from build123d import *

# Parameters (mm, degrees)
BOSS_EXTRUDE1_DEPTH = 4.5
BOSS_EXTRUDE2_START = 0.5
BOSS_EXTRUDE2_DEPTH = 0.5
FILLET1_R           = 0.5
FILLET2_R           = 0.1


with BuildPart() as part:
    # Sketch1 → Boss-Extrude1 (new body)
    with BuildSketch(Plane(origin=(0, 0, 0), x_dir=(1, 0, 0), z_dir=(0, 1, 0))):
        with BuildLine():
            Line((-2, 1.8), (2, 1.8))
            ThreePointArc((2, 1.8), (3.8, 0), (2, -1.8))
            Line((2, -1.8), (-2, -1.8))
            ThreePointArc((-2, -1.8), (-3.8, 0), (-2, 1.8))
        make_face()
    extrude(amount=BOSS_EXTRUDE1_DEPTH)

    # Sketch2 → Boss-Extrude2 (add)
    # profile 1 of 2: a face of its own
    with BuildSketch(Plane.XZ.offset(BOSS_EXTRUDE2_START)):
        with BuildLine():
            Line((-2, -2.4), (2, -2.4))
            ThreePointArc((2, -2.4), (4.4, 0), (2, 2.4))
            Line((2, 2.4), (-2, 2.4))
            ThreePointArc((-2, 2.4), (-4.4, 0), (-2, -2.4))
        make_face()
        with BuildLine():
            ThreePointArc((-2, 1.8), (-3.8, 0), (-2, -1.8))
            Line((-2, -1.8), (2, -1.8))
            ThreePointArc((2, -1.8), (3.8, 0), (2, 1.8))
            Line((2, 1.8), (-2, 1.8))
        make_face(mode=Mode.SUBTRACT)
    # profile 2 of 2: a face of its own
    with BuildSketch(Plane.XZ.offset(BOSS_EXTRUDE2_START)):
        with BuildLine():
            Line((2, 1.8), (-2, 1.8))
            ThreePointArc((-2, 1.8), (-3.8, 0), (-2, -1.8))
            Line((-2, -1.8), (2, -1.8))
            ThreePointArc((2, -1.8), (3.8, 0), (2, 1.8))
        make_face()
    extrude(amount=-BOSS_EXTRUDE2_DEPTH)

    # Fillet1
    fillet1_edges = [part.edges().sort_by_distance(p)[0] for p in [
        (3.8, 4.5, 0),
        (0, 4.5, -1.8),
        (-3.8, 4.5, 0),
        (0, 4.5, 1.8),
    ]]
    fillet(fillet1_edges, radius=FILLET1_R)

    # Fillet2
    fillet2_edges = [part.edges().sort_by_distance(p)[0] for p in [
        (0, 0, -2.4),
        (4.4, 0, 0),
        (0, 0, 2.4),
        (-4.4, 0, 0),
    ]]
    fillet(fillet2_edges, radius=FILLET2_R)


solid = part.part
Work out the finished part from the listing and answer in its coordinate system (mm). A direction names the side the tool comes from. Give positions to 0.01 mm unless a question says otherwise; leave off trailing zeros. Order: outer loops, then holes, each group sorted by start corner. A loop starts at its lowest first (then second) coordinate and runs counter-clockwise, first axis right, second up. Notation, with made-up numbers: (-33, 60) - (4, 60) arc R31 ccw to (4, 92) - close; hole circle Ø5 at (31.5, 18.25). An arc over 180 degrees is marked (long way). Answer as CSV lines item,"result". Start each with the question number.
Q1. The part is cut by section B-B (x = -1). Write down the section's boundary in (y, z), then the cut area to 3 significant figures.
Q2. The part is cut by section A-A (z = 0). Write down the section's boundary in (x, y), then the cut area to 3 significant figures.
Q3. The part is cut by section C-C (y = 2.15). Write down the section's boundary in (x, z), then the cut area to 3 significant figures.
Q4. Given pin 1 Ø3 at (x, y) = (2.5, 0) entering from -Z; pin 2 Ø3 at (x, y) = (-0.5, 2.5) entering from -Z; pin 3 Ø2 at (x, y) = (-0.5, 1.5) entering from +Z, each flat-ended and moving along its own axis, determine where each tip first touches the part or whether it passes through.
Q5. Find the intervals of material crossed by L1, parallel to Y at x = -1, z = 1.35; L2, parallel to Y at x = 3.75, z = 0.85; L3, parallel to Z at x = -2, y = 2.85, in increasing order. Write a range as [from, to].
Q6. For faces 1 (the face through (3.8, 2, 0)), 2 (the face through (0, 2, -1.8)), 3 (the face through (-3.8, 2, 0)), determine the directions among +Z, -Z, +X, -X, +Y, -Y from which every point of the face is accessible in a straight line to the end or side of a thin tool.
Check result:
1,outline,"(-0.5, -2.4) - (-0.1, -2.4) arc R0.1 ccw to (0, -2.3) - (0, -1.8) - (4, -1.8) arc R0.5 ccw to (4.5, -1.3) - (4.5, 1.3) arc R0.5 ccw to (4, 1.8) - (0, 1.8) - (0, 2.3) arc R0.1 ccw to (-0.1, 2.4) - (-0.5, 2.4) - close"
1,area,"18.5 mm²"
2,outline,"(-4.4, -0.5) - (4.4, -0.5) - (4.4, -0.1) arc R0.1 ccw to (4.3, 0) - (3.8, 0) - (3.8, 4) arc R0.5 ccw to (3.3, 4.5) - (-3.3, 4.5) arc R0.5 ccw to (-3.8, 4) - (-3.8, 0) - (-4.3, 0) arc R0.1 ccw to (-4.4, -0.1) - close"
2,area,"38.5 mm²"
3,outline,"(-2, -1.8) - (2, -1.8) arc R1.8 ccw to (2, 1.8) - (-2, 1.8) arc R1.8 ccw to start"
3,area,"24.6 mm²"
4,pin 1,"stops at z = -2.4"
4,pin 2,"stops at z = -1.8"
4,pin 3,"stops at z = 1.8"
5,L1,"y = [-0.5, 4.5]"
5,L2,"y = [-0.5, 0]"
5,L3,"z = [-1.8, 1.8]"
6,face 1,"+X, +Y"
6,face 2,"-Z, +X, -X, +Y"
6,face 3,"-X, +Y"
